Here's how the part is built. I have some questions about the finished solid (model axes, mm). Face numbers are marked on the shaded views. A direction names the side the tool comes from. Give positions to 0.01 mm unless a question says otherwise; leave off trailing zeros. Write each loop counter-clockwise with the first axis right and the second up, starting at its lowest first coordinate (ties: lowest second). Pieces come first, ordered by that corner, then holes. Notation, with made-up numbers: (29.5, 74.5) - (72.5, 74.5) arc R12 cw to (72.5, 85.5) - close; hole circle Ø3 at (-24.75, 20). An arc over 180 degrees is marked (long way). One line per item, written item: value. Start each with the question number.
1) On a 3-axis mill with a long thin cutter (end or side, diameter ignored), from which of +Z, -Z, +X, -X, +Y, -Y can I reach the whole of each face in a straight line? I mean the marked faces 4, 5 and 6. Say none if no direction works.
2) I'm going to push flat-ended pins straight in: P1, Ø0.9, axis at y = 7, z = 4.5, coming from the +X side; P2, Ø3.5, axis at y = 7.5, z = 5, coming from the -X side; P3, Ø0.5, axis at x = 17, z = 5.5, coming from the +Y side. Where does each tip first touch, or does it pass through?
3) We'd pull the mould along Z, two halves only. Please class the marked faces 1, 2 and 3: +Z half, -Z half, draft (parallel to the pull), parting line (faces both ways), or undercut.
4) Imagine slicing it at C-C on x = 17. Write out the boundary of the cut face in (y, z).
5) Please list where these lines run through material, in increasing order: L1, parallel to Z at x = 8, y = 5; L2, parallel to X at y = 7.5, z = 5.5; L3, parallel to Y at x = 14.5, z = 0. Write a range as [from, to].
6) Imagine slicing it at B-B on x = 6.75. Write out the boundary of the cut face in (y, z).
7) Imagine slicing it at A-A on x = 13.5. Write out the boundary of the cut face in (y, z).
Autodesk Inventor part; units mm, degrees
ref_plane "YZ Plane" through (0, 0, 0) normal (1, 0, 0) x (0, 1, 0)
ref_plane "XZ Plane" through (0, 0, 0) normal (0, 1, 0) x (-1, 0, 0)
ref_plane "XY Plane" through (0, 0, 0) normal (0, 0, 1) x (1, 0, 0)
sketch "Sketch1" plane through (0, 0, 0) normal (1, 0, 0) x (0, 1, 0)
  line L0 (1.5, 6.5) -> (-1.5, 6.5) construction
  line L1 (-1.5, 6.5) -> (-1.6004, 6.5) construction
  line L2 (1.5, -6.5) -> (-1.5, -6.5) construction
  line L3 (-1.5, -6.5) -> (-1.6004, -6.5) construction
  arc A0 (-1.6004, -6.5) -> (-1.6004, 6.5) centre (-14, 0) ccw
  arc A1 (1.5, -6.5) -> (1.5, 6.5) centre (-11.8333, 0) ccw
  arc A2 (1.5, -6.5) -> (1.5, 6.5) centre (-11.8333, 0) ccw
  line L4 (1.5, -6.5) -> (-1.6004, -6.5)
  line L5 (1.5, 6.5) -> (-1.6004, 6.5)
  point P0 (0, 0)
  point P1 (0, 0)
extrude "Extrusion1" add sketch "Sketch1" along normal blind 22
sketch "Sketch2" plane through (0, -1.6004, 6.5) normal (0, 0, 1) x (1, 0, 0)
  line L0 (2, 3.1004) -> (0, 3.1004)
  line L1 (2, 14.1004) -> (2, 3.1004)
  line L2 (2, 3.1004) -> (2, 14.1004)
  line L3 (16.5, 10.1004) -> (16.5, 14.1004)
  line L4 (16.5, 14.1004) -> (16.5, 10.1004)
  line L5 (16.5, 10.1004) -> (17.5, 10.1004)
  line L6 (16.5, 10.1004) -> (17.5, 10.1004)
  line L7 (17.5, 3.1004) -> (22, 3.1004)
  line L8 (17.5, 10.1004) -> (17.5, 3.1004)
  arc A0 (16.5, 14.1004) -> (2, 14.1004) centre (9.25, 14.1004) ccw
  line L9 (0, 1.6004) -> (0, 0)
  line L10 (0, 0) -> (0, 14.7425)
  line L11 (0, 3.1004) -> (0, 4.6004) construction
  line L12 (0, 3.1004) -> (-6.4438, 3.1004) construction
  line L13 (0, 3.1004) -> (6.4438, 3.1004) construction
  line L14 (2, 3.1004) -> (17.5, 3.1004)
  dimension "d2" = 180
extrude "Extrusion2" add sketch "Sketch2" against normal up to surface (13 mm away)
sketch "Sketch3" plane through (2, 1.5, 6.5) normal (-1, 0, 0) x (0, 0, 1)
  line L0 (0, 0) -> (0, -3)
  line L1 (-13, 11) -> (-13, 18.25)
  line L2 (0, 0) -> (-13, 0)
  line L3 (-13, 0) -> (-13, 18.25)
  line L4 (-13, 18.25) -> (0, 18.25)
  line L5 (0, 18.25) -> (0, 0)
  arc A0 (0, 0) -> (-13, 0) centre (-6.5, -13.3333) ccw
  arc A1 (0, 0) -> (-13, 0) centre (-6.5, -13.3333) ccw
  line L6 (-10, 1.0812) -> (-10, 7)
  line L7 (-10, 1.0812) -> (-10, 18.25)
  line L8 (-2.9979, 11) -> (-2.9979, 18.25)
  line L9 (-2.9979, 1.0807) -> (-2.9979, 18.25)
  point P0 (-6.5, -1.5)
  point P1 (-2.9979, 1.0807)
extrude "Extrusion3" cut sketch "Sketch3" against normal blind 22 contours L4 L8 L9 A0 L6 L7
fillet "Fillet1" radius 1.5 1 edges at (22, 3, 0)
fillet "Fillet2" radius 3 2 edges at (17.5, 2.1211, 5.0302) (17.5, 2.1214, -5.0291)
sketch "Sketch4" plane through (0, 0, 0) normal (0, 1, 0) x (-1, 0, 0)
  line L0 (0, 0) -> (-7.5, 0)
  line L1 (-5.5, -2) -> (-9.5, -2)
  line L2 (-9.5, -2) -> (-9.5, 2)
  line L3 (-9.5, 2) -> (-5.5, 2)
  line L4 (-5.5, 2) -> (-5.5, -2)
  dimension "d9" = 7.5
  dimension "d10" = 4
  dimension "d11" = 4
extrude "Extrusion4" add sketch "Sketch4" along normal blind 0.5 and the other way blind 1
sketch "Sketch5" plane through (0, -1, 0) normal (0, -1, 0) x (1, 0, 0)
  line L0 (9.5, 2) -> (9.5, -2)
  line L1 (5.5, -2) -> (5.5, 2)
  line L2 (9.5, -2) -> (5.5, -2)
  line L3 (5.5, -2) -> (5.5, 2)
  line L4 (5.5, 2) -> (9.5, 2)
  line L5 (9.5, 2) -> (9.5, -2)
  point P0 (0, 0)
extrude "Extrusion5" add sketch "Sketch5" along normal up to surface (0.6004 mm away)
sketch "Sketch6" plane through (5.5, -1.6004, -2) normal (0, -1, 0) x (1, 0, 0)
  line L0 (0, 4) -> (4, 4)
  line L1 (0, 0) -> (4, 0)
  line L2 (4, 0) -> (4, 4)
  line L3 (4, 4) -> (0, 4)
  line L4 (0, 4) -> (0, 0)
  point P0 (-5.5, 2)
extrude "Extrusion6" cut sketch "Sketch6" against normal blind 0.6
properties part number "Clip"
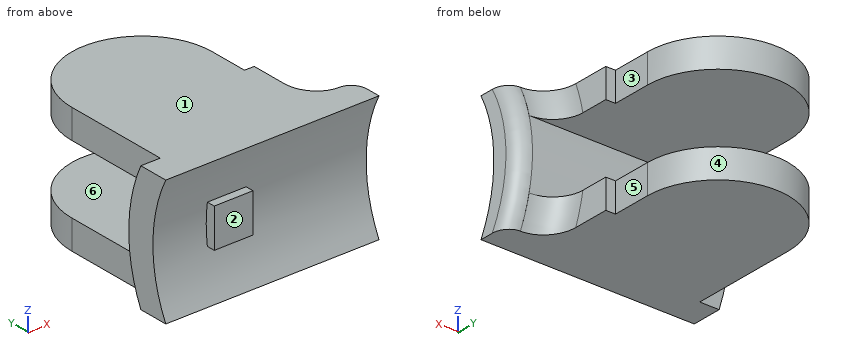
Numbers:
1. face 4: +Z, -Z, +Y
1. face 5: +Z, -Z, +X, +Y
1. face 6: +X, -X, +Y
2. P1: x = 17.5
2. P2: x = 2
2. P3: y = 8.5
3. face 1: +Z half
3. face 2: undercut
3. face 3: draft
4. outline: (-1.6, -6.5) - (8.5, -6.5) - (8.5, -3.5) - (2.58, -3.5) arc R14.83 ccw to (2.58, 3.5) - (8.5, 3.5) - (8.5, 6.5) - (-1.6, 6.5) arc R14 cw to start
5. L1: [-6.5, -3.5], [3.5, 6.5]
5. L2: [2, 17.5]
5. L3: [0, 3]
6. outline: (-1.6, -6.5) - (19.31, -6.5) - (19.31, -3.5) - (2.58, -3.5) arc R14.83 ccw to (2.58, 3.5) - (19.31, 3.5) - (19.31, 6.5) - (-1.6, 6.5) arc R14 cw to (-0.14, 2) - (-1, 2) - (-1, -2) - (-0.14, -2) arc R14 cw to start
7. outline: (-1.6, -6.5) - (18.37, -6.5) - (18.37, -3.5) - (2.58, -3.5) arc R14.83 ccw to (2.58, 3.5) - (18.37, 3.5) - (18.37, 6.5) - (-1.6, 6.5) arc R14 cw to start
